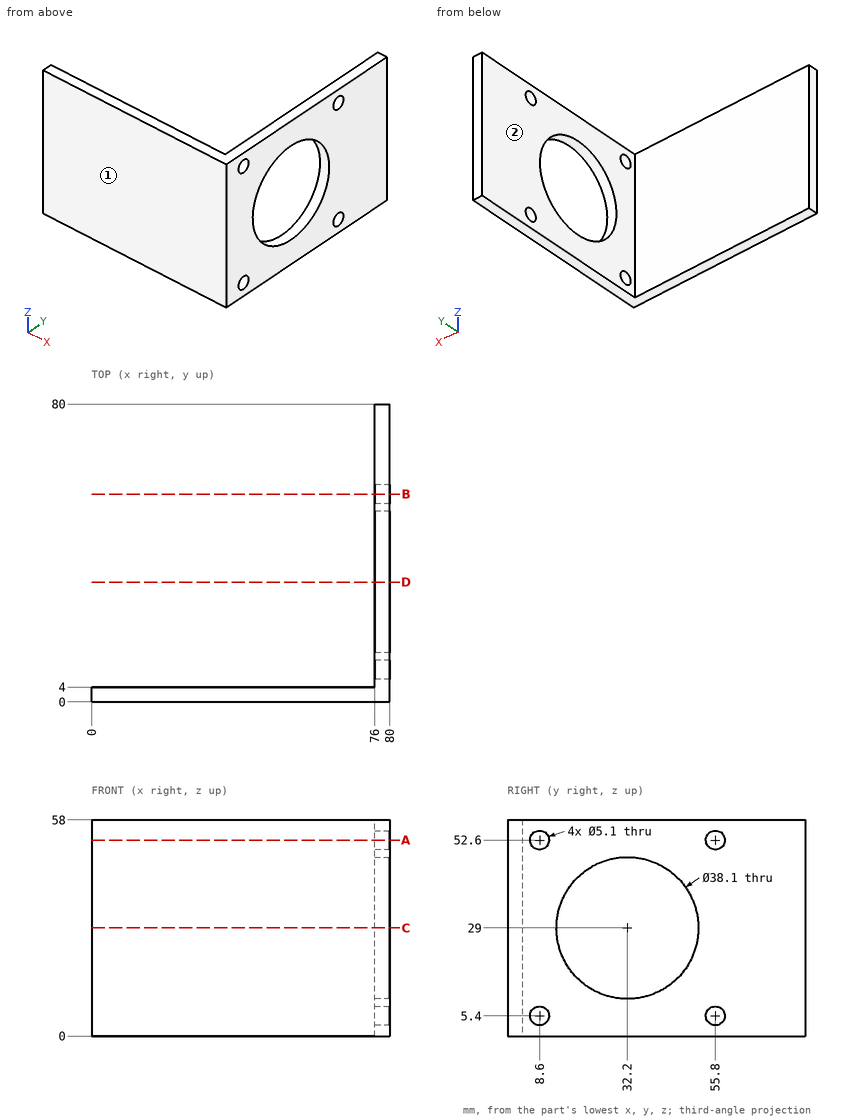
Here's the drawing with two shaded views (mm, measured from the low corner). I have some questions. A direction names the side the tool comes from. Give positions to 0.01 mm unless a question says otherwise; leave off trailing zeros. Write each loop counter-clockwise with the first axis right and the second up, starting at its lowest first coordinate (ties: lowest second). Pieces come first, ordered by that corner, then holes. Notation, with made-up numbers: (0, 79.5) -> (12, 79.5) arc R34 ccw to (12, 113.5) -> close; hole circle Ø10 at (42, 77.5). An arc over 180 degrees is marked (long way). One line per item, written item: value.
Q1. Please list where these lines run through material, in increasing order: line 1 (Y direction, x = 77.4, z = 52.6); line 2 (Z direction, x = 77, y = 8); line 3 (Z direction, x = 77, y = 32). Write a range as [from, to].
Results found:
line 1: y = [0, 6.05], [11.15, 53.25], [58.35, 80]
line 2: z = [0, 2.92], [7.88, 50.12], [55.08, 58]
line 3: z = [0, 9.95], [48.05, 58]
Q2. Imagine slicing it at D-D on y = 32.2. Please give me the cut outline in (x, z), and give its area (3 significant figures).
Results found:
outline: (76, 0) -> (80, 0) -> (80, 9.95) -> (76, 9.95) -> close; (76, 48.05) -> (80, 48.05) -> (80, 58) -> (76, 58) -> close
area: 79.6 mm^2
Q3. Which directions (+Z, -Z, +X, -X, +Y, -Y) give clear straight access to the entire face, cutting with the end or side of a thin tool? Please do the marked faces 1 and 2.
Results found:
face 1: +Z, -Z, +X, -X, -Y
face 2: +Z, -Z, -X, +Y
Q4. For P1, Ø3, axis at x = 32, z = 11.5, coming from the +Y side; P2, Ø10, axis at y = 9.5, z = 11, coming from the -X side, each with a flat end and sliding along its axis, tell me the tip position at first contact or that it passes through.
Results found:
P1: stops at y = 4
P2: stops at x = 76
Q5. Imagine slicing it at C-C on z = 29. Please give me the cut outline in (x, y), and give its area (3 significant figures).
Results found:
outline: (0, 0) -> (80, 0) -> (80, 13.15) -> (76, 13.15) -> (76, 4) -> (0, 4) -> close; (76, 51.25) -> (80, 51.25) -> (80, 80) -> (76, 80) -> close
area: 472 mm^2
Q6. Imagine slicing it at A-A on z = 52.6. Please give me the cut outline in (x, y).
Results found:
outline: (0, 0) -> (80, 0) -> (80, 6.05) -> (76, 6.05) -> (76, 4) -> (0, 4) -> close; (76, 11.15) -> (80, 11.15) -> (80, 53.25) -> (76, 53.25) -> close; (76, 58.35) -> (80, 58.35) -> (80, 80) -> (76, 80) -> close
Q7. Imagine slicing it at B-B on y = 55.8. Please give me the cut outline in (x, z), and give its area (3 significant figures).
Results found:
outline: (76, 0) -> (80, 0) -> (80, 2.85) -> (76, 2.85) -> close; (76, 7.95) -> (80, 7.95) -> (80, 50.05) -> (76, 50.05) -> close; (76, 55.15) -> (80, 55.15) -> (80, 58) -> (76, 58) -> close
area: 191 mm^2
